For this review, use the dimensioned drawing (mm, ordinates from the lowest corner) and the shaded views. A direction names the side the tool comes from. Coordinates: 2 decimals unless noted, no trailing zeros. Loops run counter-clockwise (first coordinate to the right, second up) from the corner with the lowest first, then second, coordinate; pieces in that order, holes last. Notation, with made-up numbers: (-3.5, 67.25) - (17.5, 67.25) arc R17 cw to (17.5, 86.25) - close; hole circle Ø9 at (27, 31). An arc over 180 degrees is marked (long way). Answer in a Markdown table with one row per item. Add a question column.
(1) We need section A-A on z = 12.87. Write out the cut boundary in (x, y).
(2) Machinability: for the marked faces 4, 5 and 6, which of the approach directions +Z, -Z, +X, -X, +Y, -Y give a long, thin tool a straight path to every point of the face, cutting with its end or side? Answer none if there is none.
(3) For line 1 along Y through (x, z) = (10.55, 12.87); line 2 along Y through (x, z) = (7.25, 12.87), list the stretches that pass through material, from the lowest coordinate up.
(4) For P1, Ø2, axis at x = 6, z = 23, coming from the -Y side; P2, Ø3, axis at x = 3.5, y = 22.5, coming from the -Z side; P3, Ø1, axis at x = 4, z = 20.5, coming from the -Y side, all flat-tipped, find the tip position at first contact; note any pin that passes through.
(5) Mouldability with a two-part tool opening along Y and no side actions: class the marked faces 1, 2 and 3 as +Y half, -Y half, draft (parallel to the pull), parting line (faces both ways), or undercut.
(6) We need section C-C on x = 10. Write out the cut boundary in (y, z), plus the area to 3 significant figures.
(7) We need section D-D on z = 24.25. Write out the cut boundary in (x, y).
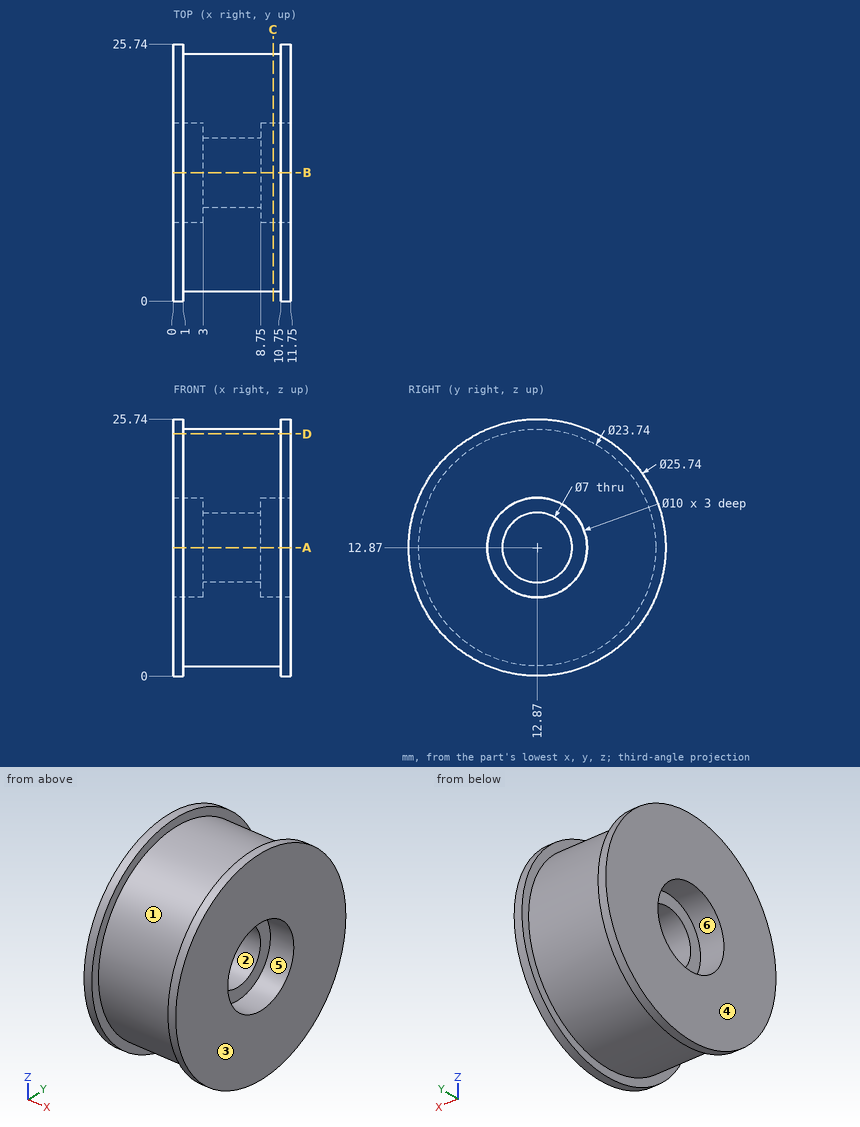
Outcome:
| question | item | result |
|---|---|---|
| 1 | outline | (0, 0) - (1, 0) - (1, 1) - (10.75, 1) - (10.75, 0) - (11.75, 0) - (11.75, 7.87) - (8.75, 7.87) - (8.75, 9.37) - (3, 9.37) - (3, 7.87) - (0, 7.87) - close; (0, 17.87) - (3, 17.87) - (3, 16.37) - (8.75, 16.37) - (8.75, 17.87) - (11.75, 17.87) - (11.75, 25.74) - (10.75, 25.74) - (10.75, 24.74) - (1, 24.74) - (1, 25.74) - (0, 25.74) - close |
| 2 | face 4 | +Z, -Z, -X, +Y, -Y |
| 2 | face 5 | +X |
| 2 | face 6 | -X |
| 3 | line 1 | 1 to 7.87, 17.87 to 24.74 |
| 3 | line 2 | 1 to 9.37, 16.37 to 24.74 |
| 4 | P1 | y = 5.28 |
| 4 | P2 | z = 4.22 |
| 4 | P3 | y = 3.38 |
| 5 | face 1 | parting line |
| 5 | face 2 | undercut |
| 5 | face 3 | draft |
| 6 | outline | circle Ø23.74 at (12.87, 12.87); hole circle Ø10 at (12.87, 12.87) |
| 6 | area | 364 mm² |
| 7 | outline | (0, 6.86) - (1, 6.86) - (1, 9.49) - (10.75, 9.49) - (10.75, 6.86) - (11.75, 6.86) - (11.75, 18.88) - (10.75, 18.88) - (10.75, 16.25) - (1, 16.25) - (1, 18.88) - (0, 18.88) - close |
